```python
from build123d import *

# Parameters (mm, degrees)
F2_R        = 1.778
F3_DEPTH    = 12.7
F5_DEPTH    = 31.75
F6_R        = 9.3599
F7_DEPTH    = 62.7888
F8_S5_R     = 9.3599
F8_T6_DEPTH = 16


# Not quite as in the source:
# - a fillet or chamfer that OpenCascade refuses, or shapes differently, is made with other operations: its cross-section is extruded or revolved along the edge and cut away or added


with BuildPart() as f1:
    # F0 (on Front) → F1 (revolve)
    with BuildSketch(Plane.XZ):
        with BuildLine():
            Line((6.35, 58.166), (0, 58.166))
            Line((0, 58.166), (0, 30.226))
            Line((0, 30.226), (0, 19.685))
            Line((0, 19.685), (0, 0))
            Line((0, 0), (0, -20.828))
            Line((0, -20.828), (7.0612, -20.828))
            Line((7.0612, -20.828), (7.0612, 0))
            Line((7.0612, 0), (7.747, 0))
            Line((7.747, 0), (8.90905, 19.685))
            add(Edge.make_bspline(
                [(8.90905, 19.685), (11.7912068963, 27.2870212793), (16.1954839903, 19.0053529362), (22.480616346, 29.8321191221), (20.828, 30.226)],
                knots=[0, 0, 0, 0, 0.5235722787, 1, 1, 1, 1], degree=3))
            Line((20.828, 30.226), (20.828, 56.896))
            add(Edge.make_bspline(
                [(15.748, 56.896), (16.993034631, 59.2658407986), (16.2821896374, 57.6469525695), (20.828, 56.896)],
                knots=[0, 0, 0, 0, 5.08, 5.08, 5.08, 5.08], degree=3))
            Line((15.748, 56.896), (7.239, 56.896))
            Line((7.239, 56.896), (7.239, 58.166))
            Line((7.239, 58.166), (6.35, 58.166))
        make_face()
    revolve(axis=Axis((0, 0, -8.4981196864), (0, 0, -1)))

    # F2 (on Front) → F3 (cut, symmetric)
    with BuildSketch(Plane.XZ):
        with Locations((0, -16.002)):
            Circle(F2_R)
    extrude(amount=F3_DEPTH, both=True, mode=Mode.SUBTRACT)

    # F4 (on Front) → F5 (join)
    with BuildSketch(Plane.XZ):
        with BuildLine():
            ThreePointArc((0, 33.7185), (7.3189087387, 36.7500912613), (10.3505, 44.069))
            ThreePointArc((10.3505, 44.069), (-7.3189087387, 51.3879087387), (0, 33.7185))
        make_face()
    extrude(amount=F5_DEPTH)

    # F6 (on face) → F7 (join)
    with BuildSketch(Plane.XZ.offset(31.75)):
        with Locations((0, 44.069)):
            Circle(F6_R)
    extrude(amount=F7_DEPTH)

    # F8: chamfer of 2.159 on 2 edges, made by hand


with BuildPart() as f8_tool2:
    # F8_s3 → F8_t4 (revolve)
    with BuildSketch(Plane.YZ):
        Polygon((-29.591, 33.7185), (-31.75, 35.8775), (-31.75, 33.7185), align=None)
    revolve(axis=Axis((0, -31.75, 44.069), (0, 1, 0)))

    # F8_s5 → F8_t6 (cut, symmetric)
    with BuildSketch(Plane.XZ.offset(30.7)):
        with Locations((0, 44.069)):
            Circle(F8_S5_R)
    extrude(amount=F8_T6_DEPTH, both=True, mode=Mode.SUBTRACT)


with BuildPart() as f1_1:
    add(f1.part)

    # F8_t1: cut F8_tool2
    add(f8_tool2.part, mode=Mode.SUBTRACT)

    # F8_s7 → F8_t8 (revolve, cut)
    with BuildSketch(Plane.XY.offset(44.069)):
        Polygon((9.3599, -92.3798), (7.2009, -94.5388), (9.3599, -94.5388), align=None)
    revolve(axis=Axis((0, -94.5388, 44.069), (0, -1, 0)), mode=Mode.SUBTRACT)

    # F9: fillet of radius 1.651 on 2 edges, made by hand

    # F9_s1 → F9_t2 (revolve, cut)
    with BuildSketch(Plane.XZ):
        with BuildLine():
            ThreePointArc((7.239, 56.896), (6.6564696827, 57.8101509565), (5.6325629486, 58.166))
            Line((5.6325629486, 58.166), (5.6325629486, 58.19902))
            Line((5.6325629486, 58.19902), (7.239, 58.19902))
            Line((7.239, 58.19902), (7.27202, 58.166))
            ThreePointArc((7.27202, 58.166), (7.27202, 57.531), (7.271128741, 56.90362))
            Line((7.271128741, 56.90362), (7.239, 56.896))
        make_face()
    revolve(axis=Axis((0, 0, 58.166), (0, 0, -1)), mode=Mode.SUBTRACT)

    # F9_s3 → F9_t4 (revolve)
    with BuildSketch(Plane.XZ):
        with BuildLine():
            ThreePointArc((21.1597456512, 30.0175911775), (20.9131312427, 30.4869361434), (20.828, 31.010248703))
            Line((20.828, 31.010248703), (20.79498, 31.010248703))
            Line((20.79498, 31.010248703), (20.79498, 30.226))
            Line((20.79498, 30.226), (20.8203445184, 30.1938796949))
            ThreePointArc((20.8203445184, 30.1938796949), (20.9949538129, 30.1235602191), (21.1333605642, 29.997738027))
            Line((21.1333605642, 29.997738027), (21.1597456512, 30.0175911775))
        make_face()
    revolve(axis=Axis((0, 0, 30.226), (0, 0, -1)))


solid = f1_1.part
```
Here's how the part is built. I have some questions about the finished solid (model axes, mm). A direction names the side the tool comes from. Round coordinates to 2 decimals unless told otherwise and drop trailing zeros. Write each loop counter-clockwise with the first axis right and the second up, starting at its lowest first coordinate (ties: lowest second). Pieces come first, ordered by that corner, then holes.
Q1. If we mould it in two halves opening along X, with no side actions, what happens to faces 1 (the flat face through (7, 3, 56.896)), 2 (the flat face through (0, 0, 58.166)), 3 (the cylindrical face through (3.258, 6.264, -10.268))? For each: +X half, -X half, draft (parallel to the pull), parting line (faces both ways), or undercut.
Q2. If we section it at B-B on z = 16.5: Write out the boundary of the cut face in (x, y), plus the area to 3 significant figures.
Q3. If we section it at A-A on y = -60: Write out the boundary of the cut face in (x, z), plus the area to 3 significant figures.
Q4. Will these pins go through, and if not, where does the flat tip stop? P1, Ø6, axis at x = 6, z = 14, coming from the +Y side; P2, Ø10, axis at x = 15.5, z = 46.5, coming from the -Y side; P3, Ø4, axis at x = -6, z = 22, coming from the -Y side.
Q5. Which directions (+Z, -Z, +X, -X, +Y, -Y) give clear straight access to the entire face, cutting with the end or side of a thin tool? Please do faces 4 (the flat face through (-7, -2, 0)), 5 (the cylindrical face through (-2.03, -61.91, 34.93)), 6 (the flat face through (0, -94.539, 44)).
Q6. Please list where these lines run through material, in increasing order: probe 1 along Z at (x, y) = (0, -2); probe 2 along Y at (x, z) = (-3, 18.5); probe 3 along Z at (x, y) = (5, -25).
Answer below:
1. face 1: undercut
1. face 2: draft
1. face 3: parting line
2. outline: circle Ø17.44 at (0, 0)
2. area: 239 mm2
3. outline: circle Ø18.72 at (0, 44.07)
3. area: 275 mm2
4. P1: stops at y = 8.05
4. P2: stops at y = -17.99
4. P3: stops at y = -16.27
5. face 4: -Z
5. face 5: -Y
5. face 6: +Z, -Z, +X, -X, -Y
6. probe 1: z = -20.83 to -17.78, -14.22 to 58.17
6. probe 2: y = -8.31 to 8.31
6. probe 3: z = 35.01 to 53.13
